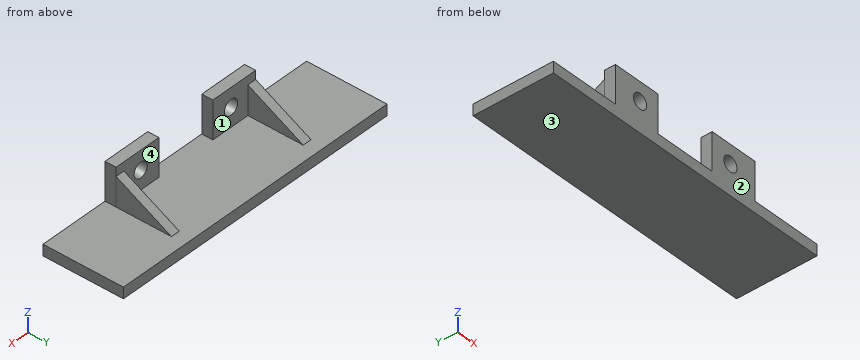
```python
from build123d import *

# Parameters (mm, degrees)
SKETCH1_W           = 86
SKETCH1_H           = 23
BOSS_EXTRUDE1_DEPTH = 3.175
BOSS_EXTRUDE2_DEPTH = 3.175
RIB4_REACH          = 68.401
SKETCH11_WALL_W     = 152.68434621
SKETCH11_WALL_H     = 2.54
SKETCH17_W          = 11.43
SKETCH17_H          = 10.795
CUT_EXTRUDE1_DEPTH  = 127
SKETCH18_R          = 2.159
CUT_EXTRUDE2_DEPTH  = 127


with BuildPart() as part:
    # Sketch1 → Boss-Extrude1 (new body)
    with BuildSketch(Plane.XY):
        Rectangle(SKETCH1_W, SKETCH1_H)
    extrude(amount=-BOSS_EXTRUDE1_DEPTH)

    # Sketch3 → Boss-Extrude2 (add)
    with BuildSketch(Plane(origin=(0, -11.5, 0), x_dir=(-1, 0, 0), z_dir=(0, -1, 0))):
        Polygon((34.200000011, 0), (34.200000011, -10.795), (8.80000001, -10.795), (8.800000011, 0), align=None)
        Polygon((-34.200000011, 0), (-34.200000011, -10.795), (-8.80000001, -10.795), (-8.800000011, 0), align=None)
    extrude(amount=-BOSS_EXTRUDE2_DEPTH)

    # Sketch11 wall → Rib4 (add, up to next)
    with BuildSketch(Plane(origin=(-21.500000011, -0.407189587, 4.154640606), x_dir=(-5.6e-11, -0.885499596527, 0.46464014522), z_dir=(0, 0.46464014522, 0.885499596527)), mode=Mode.PRIVATE) as rib4_sk1:
        Rectangle(SKETCH11_WALL_W, SKETCH11_WALL_H)
    rib4_tool1 = extrude(rib4_sk1.sketch, amount=-RIB4_REACH, mode=Mode.PRIVATE) - part.part
    rib4 = rib4_tool1.solids().sort_by_distance((-21.500000011, -0.407189587, 4.154640606))[0]
    add(rib4)

    # Mirror1: Rib4 across plane
    add(rib4.mirror(Plane(origin=(0, 0, 0), x_dir=(0, 0, 1), z_dir=(1, 0, 0))))

    # Sketch17 → Cut-Extrude1 (cut)
    with BuildSketch(Plane(origin=(0, 11.5, 0), x_dir=(1, 0, 0), z_dir=(0, 1, 0))):
        with Locations((-28.485000011, -5.3975)):
            Rectangle(SKETCH17_W, SKETCH17_H)
    cut_extrude1 = extrude(amount=-CUT_EXTRUDE1_DEPTH, mode=Mode.SUBTRACT)

    # Mirror2: Cut-Extrude1 across plane
    add(cut_extrude1.mirror(Plane(origin=(0, 0, 0), x_dir=(0, 0, 1), z_dir=(1, 0, 0))), mode=Mode.SUBTRACT)

    # Sketch18 → Cut-Extrude2 (cut)
    with BuildSketch(Plane(origin=(0, 11.5, 0), x_dir=(1, 0, 0), z_dir=(0, 1, 0))):
        with Locations(Location((-14.74281704, -5.421760778, 0), (0, 0, 270))):
            Circle(SKETCH18_R)
    cut_extrude2 = extrude(amount=-CUT_EXTRUDE2_DEPTH, mode=Mode.SUBTRACT)

    # Mirror3: Cut-Extrude2 across plane
    add(cut_extrude2.mirror(Plane(origin=(0, 0, 0), x_dir=(0, 0, 1), z_dir=(1, 0, 0))), mode=Mode.SUBTRACT)


solid = part.part
```
Verification items for the finished model (mm, model axes). Face numbers are marked on the shaded views. A direction names the side the tool comes from. Give positions to 0.01 mm unless a question says otherwise; leave off trailing zeros. Loops run counter-clockwise (first coordinate to the right, second up) from the corner with the lowest first, then second, coordinate; pieces in that order, holes last. Notation, with made-up numbers: M 47,-17 L 52,-17 A29 ccw 52,5 Z; hole C 45.25,28 d10. An arc over 180 degrees is marked long. Return JSON: item names as keys, results as strings.
1) Tool access check on the marked faces 1 and 2. Record the directions out of +Z, -Z, +X, -X, +Y, -Y that give a thin tool (end or side, any length) a straight path to the whole face; none if there is none.
Findings:
{"face 1": "+Z, +Y", "face 2": "+Z, -Z, +X, -X, -Y"}
2) Section check C-C, the plane z = 6.5. Enter the section's corners in (x, y) (3 decimals), and give its area (3 significant figures).
Findings:
{"outline": "M -22.77,-11.5 L -16.613,-11.5 L -16.613,-8.325 L -20.23,-8.325 L -20.23,-4.877 L -22.77,-4.877 Z; M -12.872,-11.5 L -8.8,-11.5 L -8.8,-8.325 L -12.872,-8.325 Z; M 8.8,-11.5 L 12.872,-11.5 L 12.872,-8.325 L 8.8,-8.325 Z; M 16.613,-11.5 L 22.77,-11.5 L 22.77,-4.877 L 20.23,-4.877 L 20.23,-8.325 L 16.613,-8.325 Z", "area": "82.5 mm2"}
3) Section check A-A, the plane z = 1.5. Enter the section's corners in (x, y) (3 decimals), and give its area (3 significant figures).
Findings:
{"outline": "M -22.77,-11.5 L -8.8,-11.5 L -8.8,-8.325 L -20.23,-8.325 L -20.23,4.652 L -22.77,4.652 Z; M 8.8,-11.5 L 22.77,-11.5 L 22.77,4.652 L 20.23,4.652 L 20.23,-8.325 L 8.8,-8.325 Z", "area": "155 mm2"}
4) Mould release check, pull along X, two halves, no side actions. Record for the marked faces 3 and 4: released by +X, released by -X, zero draft, split by the parting line, or undercut.
Findings:
{"face 3": "zero draft", "face 4": "undercut"}
5) Section check D-D, the plane y = -5. Enter the section's corners in (x, z) (3 decimals).
Findings:
{"outline": "M -43,-3.175 L 43,-3.175 L 43,0 L 22.77,0 L 22.77,6.565 L 20.23,6.565 L 20.23,0 L -20.23,0 L -20.23,6.565 L -22.77,6.565 L -22.77,0 L -43,0 Z"}
6) Material ranges on L1, parallel to X at y = -8.25, z = 2; L2, parallel to X at y = -9.75, z = 1.25; L3, parallel to Z at x = 28, y = -8.75 (3 decimals), recorded low to high. Write a range as [from, to].
Findings:
{"L1": "x = [-22.77, -20.23], [20.23, 22.77]", "L2": "x = [-22.77, -8.8], [8.8, 22.77]", "L3": "z = [-3.175, 0]"}
7) Gauge pin test, flat ends, axial feed: P1, Ø1, axis at y = -9.5, z = 6.5, coming from the +X side; P2, Ø1, axis at y = 0.5, z = 5, coming from the +X side; P3, Ø1, axis at y = -10, z = 3, coming from the -X side; P4, Ø8, axis at x = 12, z = 6.5, coming from the +Y side (3 decimals). Record the tip position at first contact, or that the pin passes through.
Findings:
{"P1": "stops at x = 22.77", "P2": "passes through", "P3": "stops at x = -22.77", "P4": "stops at y = -8.325"}
8) Section check B-B, the plane y = -9.5. Enter the section's corners in (x, z) (3 decimals), and give its area (3 significant figures).
Findings:
{"outline": "M -43,-3.175 L 43,-3.175 L 43,0 L 22.77,0 L 22.77,10.795 L 8.8,10.795 L 8.8,0 L -8.8,0 L -8.8,10.795 L -22.77,10.795 L -22.77,0 L -43,0 Z; hole C -14.743,5.422 d4.318; hole C 14.743,5.422 d4.318", "area": "545 mm2"}
